```python
from build123d import *

# Parameters (mm, degrees)
SKETCH1_R               = 5
SKETCH1_R_2             = 31.5
BOSS_EXTRUDE1_DEPTH     = 21
CUT_EXTRUDE1_DEPTH      = 249.276960573
CUT_EXTRUDE1_DEPTH_BACK = 249.276960573
SKETCH1_3_R             = 17.5
SKETCH1_3_R_2           = 12
BOSS_EXTRUDE2_DEPTH     = 21
SKETCH1_4_R             = 31.5
SKETCH1_4_R_2           = 26
BOSS_EXTRUDE3_DEPTH     = 35
CUT_EXTRUDE2_START      = 2.5
CUT_EXTRUDE2_DEPTH      = 70
CUT_EXTRUDE3_DEPTH      = 14


with BuildPart() as part:
    # Sketch1 → Boss-Extrude1 (new, symmetric)
    with BuildSketch(Plane(origin=(0, 0, 0), x_dir=(1, 0, 0), z_dir=(0, 1, 0))):
        with BuildLine():
            Line((221.187786225, 9.494895459), (88.904140781, 13.002249852))
            ThreePointArc((88.904140781, 13.002249852), (53.309733953, 23.515221578), (27.680495601, 50.35970916))
            ThreePointArc((27.680495601, 50.35970916), (18.1834351, 56.969515961), (7.179772337, 53.391372602))
            ThreePointArc((7.179772337, 53.391372602), (-14.863061383, 42.091119402), (-39.431134928, 38.930106423))
            ThreePointArc((-39.431134928, 38.930106423), (-49.321982863, 35.019426592), (-52.982993526, 25.033471929))
            ThreePointArc((-52.982993526, 25.033471929), (-48.490958117, 0), (-52.982993526, -25.033471929))
            ThreePointArc((-52.982993526, -25.033471929), (-49.321982863, -35.019426592), (-39.431134928, -38.930106423))
            ThreePointArc((-39.431134928, -38.930106423), (-14.863061383, -42.091119402), (7.179772337, -53.391372602))
            ThreePointArc((7.179772337, -53.391372602), (18.1834351, -56.969515961), (27.680495601, -50.35970916))
            ThreePointArc((27.680495601, -50.35970916), (53.309733953, -23.515221578), (88.904140781, -13.002249852))
            Line((88.904140781, -13.002249852), (221.187786225, -9.494895459))
            ThreePointArc((221.187786225, -9.494895459), (231.340206045, -10.720138116), (240.705148821, -14.827533226))
            ThreePointArc((240.705148821, -14.827533226), (232.5, 0), (240.705148821, 14.827533226))
            ThreePointArc((240.705148821, 14.827533226), (231.340206045, 10.720138116), (221.187786225, 9.494895459))
        make_face()
        with Locations(Location((15, -43, 0), (0, 0, 90))):
            Circle(SKETCH1_R, mode=Mode.SUBTRACT)
        with Locations(Location((-40, -26, 0), (0, 0, 90))):
            Circle(SKETCH1_R, mode=Mode.SUBTRACT)
        with Locations(Location((0, 0, 0), (0, 0, 90))):
            Circle(SKETCH1_R_2, mode=Mode.SUBTRACT)
        with Locations(Location((-40, 26, 0), (0, 0, 90))):
            Circle(SKETCH1_R, mode=Mode.SUBTRACT)
        with Locations(Location((15, 43, 0), (0, 0, 90))):
            Circle(SKETCH1_R, mode=Mode.SUBTRACT)
    extrude(amount=BOSS_EXTRUDE1_DEPTH, both=True)

    # Sketch2 → Cut-Extrude1 (cut, two sides: drawn at the far end of the back side and taken through both)
    with BuildSketch(Plane.XY.offset(-CUT_EXTRUDE1_DEPTH_BACK)):
        with BuildLine():
            Line((240.705148821, 21), (221.187786225, 21))
            Line((221.187786225, 21), (88.904140781, 21))
            ThreePointArc((88.904140781, 21), (106.542213745, 14.283423215), (125.27720774, 12))
            Line((125.27720774, 12), (240.705148821, 12))
            Line((240.705148821, 12), (240.705148821, 21))
        make_face()
        with BuildLine():
            Line((240.705148821, -12), (125.27720774, -12))
            ThreePointArc((125.27720774, -12), (106.542213745, -14.283423215), (88.904140781, -21))
            Line((88.904140781, -21), (221.187786225, -21))
            Line((221.187786225, -21), (240.705148821, -21))
            Line((240.705148821, -21), (240.705148821, -12))
        make_face()
    extrude(amount=CUT_EXTRUDE1_DEPTH + CUT_EXTRUDE1_DEPTH_BACK, mode=Mode.SUBTRACT)

    # Sketch1_3 → Boss-Extrude2 (add, symmetric)
    with BuildSketch(Plane(origin=(0, 0, 0), x_dir=(1, 0, 0), z_dir=(0, 1, 0))):
        with Locations(Location((250, 0, 0), (0, 0, 270))):
            Circle(SKETCH1_3_R)
        with Locations(Location((250, 0, 0), (0, 0, 90))):
            Circle(SKETCH1_3_R_2, mode=Mode.SUBTRACT)
    extrude(amount=BOSS_EXTRUDE2_DEPTH, both=True)

    # Sketch1_4 → Boss-Extrude3 (add, symmetric)
    with BuildSketch(Plane(origin=(0, 0, 0), x_dir=(1, 0, 0), z_dir=(0, 1, 0))):
        with Locations(Location((0, 0, 0), (0, 0, 270))):
            Circle(SKETCH1_4_R)
        with Locations(Location((0, 0, 0), (0, 0, 270))):
            Circle(SKETCH1_4_R_2, mode=Mode.SUBTRACT)
    extrude(amount=BOSS_EXTRUDE3_DEPTH, both=True)

    # Sketch1_5 → Cut-Extrude2 (cut)
    with BuildSketch(Plane(origin=(0, 0, 0), x_dir=(1, 0, 0), z_dir=(0, 1, 0)).offset(CUT_EXTRUDE2_START)):
        with BuildLine():
            Line((70, -6), (220, -6))
            ThreePointArc((220, -6), (226, 0), (220, 6))
            Line((220, 6), (70, 6))
            ThreePointArc((70, 6), (64, 0), (70, -6))
        make_face()
    cut_extrude2 = extrude(amount=CUT_EXTRUDE2_DEPTH, mode=Mode.SUBTRACT)

    # Mirror1: Cut-Extrude2 across plane
    add(cut_extrude2.mirror(Plane.ZX), mode=Mode.SUBTRACT)

    # Sketch5 → Cut-Extrude3 (cut, symmetric)
    with BuildSketch(Plane(origin=(0, 0, 0), x_dir=(1, 0, 0), z_dir=(0, 1, 0))):
        with BuildLine():
            ThreePointArc((88.904140781, 13.002249852), (49.66976816, 17.602087151), (11.897396977, 29.16679525))
            ThreePointArc((11.897396977, 29.16679525), (-31.5, 0), (11.897396977, -29.16679525))
            ThreePointArc((11.897396977, -29.16679525), (49.66976816, -17.602087151), (88.904140781, -13.002249852))
            ThreePointArc((88.904140781, -13.002249852), (53.309733953, -23.515221578), (27.680495601, -50.35970916))
            ThreePointArc((27.680495601, -50.35970916), (18.1834351, -56.969515961), (7.179772337, -53.391372602))
            ThreePointArc((7.179772337, -53.391372602), (-14.863061383, -42.091119402), (-39.431134928, -38.930106423))
            ThreePointArc((-39.431134928, -38.930106423), (-49.321982863, -35.019426592), (-52.982993526, -25.033471929))
            ThreePointArc((-52.982993526, -25.033471929), (-48.490958117, 0), (-52.982993526, 25.033471929))
            ThreePointArc((-52.982993526, 25.033471929), (-49.321982863, 35.019426592), (-39.431134928, 38.930106423))
            ThreePointArc((-39.431134928, 38.930106423), (-14.863061383, 42.091119402), (7.179772337, 53.391372602))
            ThreePointArc((7.179772337, 53.391372602), (18.1834351, 56.969515961), (27.680495601, 50.35970916))
            ThreePointArc((27.680495601, 50.35970916), (53.309733953, 23.515221578), (88.904140781, 13.002249852))
        make_face()
    extrude(amount=CUT_EXTRUDE3_DEPTH, both=True, mode=Mode.SUBTRACT)


solid = part.part
```
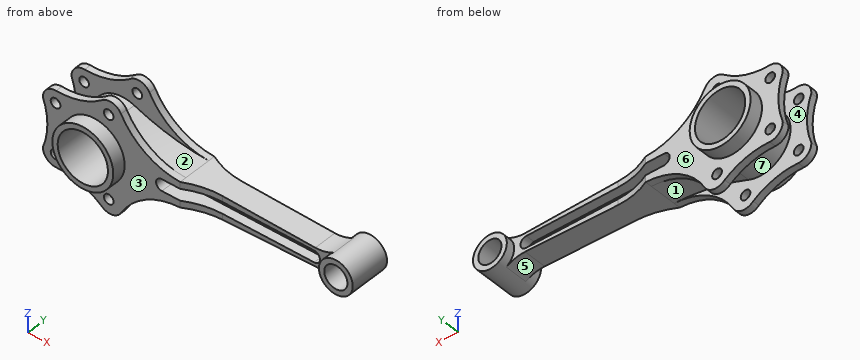
Design review of the part built by this model. Coordinates are the model's own, in mm. Face numbers are marked on the shaded views. A direction names the side the tool comes from. Give positions to 0.01 mm unless a question says otherwise; leave off trailing zeros. Write each loop counter-clockwise with the first axis right and the second up, starting at its lowest first coordinate (ties: lowest second). Pieces come first, ordered by that corner, then holes. Notation, with made-up numbers: (-8.75, 82) -> (48.25, 82) arc R6 cw to (48.25, 93) -> close; hole circle Ø6 at (34.25, 71.5). An arc over 180 degrees is marked (long way). Answer in a Markdown table with one row per item.
(1) For the marked faces 1, 2, 3 and 4, list the 3-axis set-ups (+Z, -Z, +X, -X, +Y, -Y) from which the entire face can be reached by the end or side of a thin tool; tool diameter is ignored.
Results:
| item | result |
|---|---|
| face 1 | -Z |
| face 2 | +Z |
| face 3 | -Y |
| face 4 | none |
(2) Consider section D-D (z = 0). Count the separate pieces of the cut face and the enclosed holes in it, then the cut area to 3 significant figures.
Results:
| item | result |
|---|---|
| separate pieces | 3 |
| enclosed holes | 0 |
| area | 3,800 mm2 |
(3) Consider section C-C (x = 195.5). State the section outline as (y, z) points.
Results:
| item | result |
|---|---|
| outline | (-12, -10.18) -> (12, -10.18) -> (12, -6) -> (2.5, -6) -> (2.5, 6) -> (12, 6) -> (12, 10.18) -> (-12, 10.18) -> (-12, 6) -> (-2.5, 6) -> (-2.5, -6) -> (-12, -6) -> close |
(4) Clearance check with flat-ended pins moving along their axes: pin 1 (13 mm diameter, centred on x = 128.5, z = 2.5, fed in from -Y); pin 2 (3 mm diameter, centred on y = -17, z = 45, fed in from +X); pin 3 (10 mm diameter, centred on x = 23.5, y = -13, fed in from +Z); pin 4 (14.5 mm diameter, centred on x = 250, z = 0, fed in from -Y). State where each tip first meets the part, or that it passes through.
Results:
| item | result |
|---|---|
| pin 1 | y = -12.03 |
| pin 2 | x = 31.96 |
| pin 3 | z = 56.9 |
| pin 4 | through |
(5) Consider section A-A (x = 0). State the section outline as (y, z) points, then the cut area to 3 significant figures.
Results:
| item | result |
|---|---|
| outline | (-35, -31.5) -> (-21, -31.5) -> (-21, -48.62) -> (-14, -48.62) -> (-14, -31.5) -> (14, -31.5) -> (14, -48.62) -> (21, -48.62) -> (21, -31.5) -> (35, -31.5) -> (35, -26) -> (-35, -26) -> close; (-35, 26) -> (35, 26) -> (35, 31.5) -> (21, 31.5) -> (21, 48.62) -> (14, 48.62) -> (14, 31.5) -> (-14, 31.5) -> (-14, 48.62) -> (-21, 48.62) -> (-21, 31.5) -> (-35, 31.5) -> close |
| area | 1,250 mm2 |
(6) To check wall thickness, follow probe 1 along Z at (x, y) = (-40, 18); probe 2 along X at (y, z) = (-1.5, 0); probe 3 along X at (y, z) = (-3, 0). State the ranges of each line that lie inside material, in increasing order.
Results:
| item | result |
|---|---|
| probe 1 | -38.94 to -31, -21 to 21, 31 to 38.94 |
| probe 2 | -31.5 to -26, 26 to 238, 262 to 267.5 |
| probe 3 | -31.5 to -26, 26 to 64, 226 to 238, 262 to 267.5 |
(7) Consider section B-B (z = 43). State the section outline as (x, y) points.
Results:
| item | result |
|---|---|
| outline | (-12.13, -21) -> (10, -21) -> (10, -14) -> (-12.13, -14) -> close; (-12.13, 14) -> (10, 14) -> (10, 21) -> (-12.13, 21) -> close; (20, -21) -> (32.32, -21) -> (32.32, -14) -> (20, -14) -> close; (20, 14) -> (32.32, 14) -> (32.32, 21) -> (20, 21) -> close |
(8) Mouldability with a two-part tool opening along Y and no side actions: class the marked faces 5, 6 and 7 as +Y half, -Y half, draft (parallel to the pull), parting line (faces both ways), or undercut.
Results:
| item | result |
|---|---|
| face 5 | draft |
| face 6 | +Y half |
| face 7 | undercut |
